Read the model definition and answer for the solid it produces. Units are mm, in the model's axes. A direction names the side the tool comes from. Coordinates: 2 decimals unless noted, no trailing zeros. Write each loop counter-clockwise with the first axis right and the second up, starting at its lowest first coordinate (ties: lowest second). Pieces come first, ordered by that corner, then holes. Notation, with made-up numbers: (-18, 13) -> (-13, 13) arc R10 ccw to (-13, 24) -> close; hole circle Ø3 at (40, 57.5). An arc over 180 degrees is marked (long way). Answer in a Markdown table with one row per item. Add a question column.
Item 1: Given pin 1 Ø2 at (x, y) = (0, 0) entering from +Z; pin 2 Ø4 at (y, z) = (-10.5, 16) entering from +X; pin 3 Ø2 at (x, z) = (-5.5, 26.5) entering from +Y, each flat-ended and moving along its own axis, determine where each tip first touches the part or whether it passes through.
Item 2: Section D-D on y = -9 is taken. Write down the section's boundary in (x, z), then the cut area to 3 significant figures.
Item 3: Section C-C on z = 37 is taken. Write down the section's boundary in (x, y).
Item 4: Which of the six approach directions +Z, -Z, +X, -X, +Y, -Y give full straight-line access (tool end or side, diameter ignored) to faces 1 (the face through (-3.36, -0.44, 12.68)), 2 (the face through (-3.36, 0.44, 52.32)), 3 (the face through (0, 4, 65))?
Item 5: For a pull along X with two mould halves and no side action, classify faces 4 (the face through (0, 4, 0)), 5 (the face through (-14.985, -0.66, 32.045)), 6 (the face through (0, 0, 25)) as +X half, -X half, draft (parallel to the pull), parting line (faces both ways), or undercut.
Item 6: Section A-A on y = 0 is taken. Write down the section's boundary in (x, z), then the cut area to 3 significant figures.
Item 7: Straight lines are drawn through the part: line 1 (Y direction, x = 0, z = 51.5); line 2 (Y direction, x = -1.75, z = 55); line 3 (X direction, y = 2, z = 55). For each, find the intervals that lie inside material, in ascending order. Write a range as from..to.
Autodesk Fusion 360 part; units mm, degrees
sketch "Sketch1" plane through (0, 0, 0) normal (0, 0, 1) x (1, 0, 0)
  circle A0 centre (0, 0) radius 15
  dimension "d1" = 30
extrude "Extrude1" add sketch "Sketch1" along normal blind 65
hole "Hole1" at (0, 0, 65) direction (0, 0, -1) diameter 6.78 depth 25 tip angle 180
hole "Hole2" at (0, 0, 0) direction (0, 0, 1) diameter 6.78 depth 25 tip angle 180
Results below:
| question | item | result |
|---|---|---|
| 1 | pin 1 | stops at z = 40 |
| 1 | pin 2 | stops at x = 12.36 |
| 1 | pin 3 | stops at y = 14.31 |
| 2 | outline | (-12, 0) -> (12, 0) -> (12, 65) -> (-12, 65) -> close |
| 2 | area | 1,560 mm2 |
| 3 | outline | circle Ø30 at (0, 0) |
| 4 | face 1 | -Z |
| 4 | face 2 | +Z |
| 4 | face 3 | +Z, +X, -X, +Y, -Y |
| 5 | face 4 | draft |
| 5 | face 5 | parting line |
| 5 | face 6 | undercut |
| 6 | outline | (-15, 0) -> (-3.39, 0) -> (-3.39, 25) -> (3.39, 25) -> (3.39, 0) -> (15, 0) -> (15, 65) -> (3.39, 65) -> (3.39, 40) -> (-3.39, 40) -> (-3.39, 65) -> (-15, 65) -> close |
| 6 | area | 1,610 mm2 |
| 7 | line 1 | y = -15..-3.39, 3.39..15 |
| 7 | line 2 | y = -14.9..-2.9, 2.9..14.9 |
| 7 | line 3 | x = -14.87..-2.74, 2.74..14.87 |
